from build123d import *

# Parameters (mm, degrees)
F1_DEPTH = 25
F2_SIZE2 = 55.99999
F2_SIZE  = 17.49999


# Not quite as in the source:
# - a fillet or chamfer is up to 0.001 mm smaller than in the source, because OpenCascade refuses the exact size


with BuildPart() as f1:
    # F0 (on Front) → F1 (new body, symmetric)
    with BuildSketch(Plane.XZ):
        Polygon((25, -29.9881670944), (7.5, 26.0118329056), (-7.5, 26.0118329056), (-25, -29.9881670944), align=None)
    extrude(amount=F1_DEPTH, both=True)

    # F2 (size 17.5 and 56 in the source; OpenCascade refuses exactly that, so slightly less here)
    f2_edges = [f1.edges().sort_by_distance(p)[0] for p in [
        (0, 25, 26.011833),
        (0, -25, 26.011833),
    ]]
    f2_side = f1.faces().sort_by_distance((0, 0, 26.011833))[0]
    chamfer(f2_edges, length=F2_SIZE, length2=F2_SIZE2, reference=f2_side)


solid = f1.part
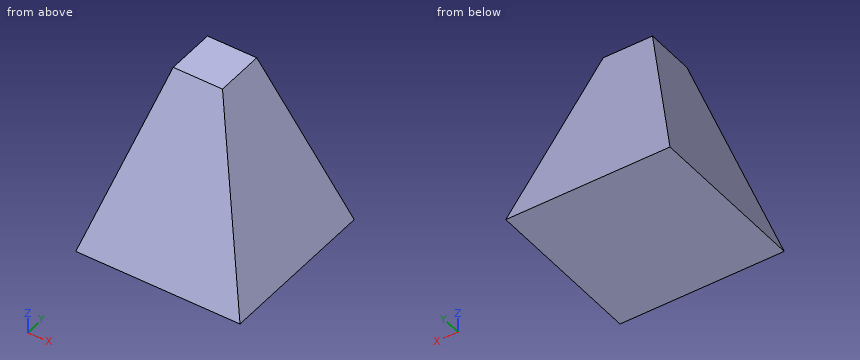
CAD build for the part. Positions are in the model's coordinates, mm. Round coordinates to 2 decimals unless told otherwise and drop trailing zeros. Write each loop counter-clockwise with the first axis right and the second up, starting at its lowest first coordinate (ties: lowest second). Pieces come first, ordered by that corner, then holes. Notation, with made-up numbers: M 78,-6 L 84,-6 A26 cw 84,15 Z; hole C -4.75,14.5 d6. An arc over 180 degrees is marked long. Use a Markdown table: item, result. Add a question column.
1. Drill centre lines: probe 1 along X at (y, z) = (10.5, -20.5); probe 2 along Y at (x, z) = (14, -24); probe 3 along X at (y, z) = (-6, -22). Where is each one in solid material? Low to high.
2. Flat gauge pins, fed straight in: P1, Ø1.5, axis at x = 17, z = -15.5, coming from the -Y side; P2, Ø6, axis at y = 5.5, z = -21, coming from the +X side; P3, Ø10, axis at x = -19, z = 15, coming from the +Y side. Where does each tip first touch, or does it go through?
3. Slice it at B-B on y = -14. Give the cut face in (x, z).
4. Slice it at C-C on z = -7. Give the cut face in (x, y), then the cut area to 3 significant figures.
Reply:
| question | item | result |
|---|---|---|
| 1 | probe 1 | x = -22.03 to 22.03 |
| 1 | probe 2 | y = -23.13 to 23.13 |
| 1 | probe 3 | x = -22.5 to 22.5 |
| 2 | P1 | stops at y = -20.71 |
| 2 | P2 | stops at x = 23.13 |
| 2 | P3 | passes through |
| 3 | outline | M -25,-29.99 L 25,-29.99 L 14,5.21 L -14,5.21 Z |
| 4 | outline | M -17.82,-17.82 L 17.82,-17.82 L 17.82,17.82 L -17.82,17.82 Z |
| 4 | area | 1,270 mm^2 |
